Could you check a few things on this model? Use its own coordinates, in mm. Face numbers are marked on the shaded views. A direction names the side the tool comes from. Coordinates: 2 decimals unless noted, no trailing zeros. Write each loop counter-clockwise with the first axis right and the second up, starting at its lowest first coordinate (ties: lowest second). Pieces come first, ordered by that corner, then holes.
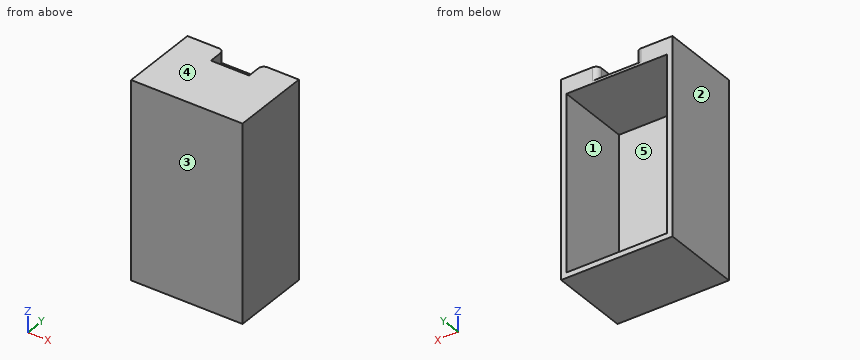
```python
from build123d import *

# Parameters (mm, degrees)
ESQUISSE1_W             = 210
ESQUISSE1_H             = 150
BOSS_EXTRU_1_DEPTH      = 370
ESQUISSE2_W             = 190
ESQUISSE2_H             = 330
ENL_V_MAT_EXTRU_1_DEPTH = 140
ESQUISSE6_W             = 72
ESQUISSE6_H             = 25
ENL_V_MAT_EXTRU_4_DEPTH = 35
ESQUISSE7_W             = 72
ESQUISSE7_H             = 20
ENL_V_MAT_EXTRU_5_DEPTH = 15
CONG_3_R                = 10
CONG_4_R                = 10
CONG_5_R                = 10


with BuildPart() as part:
    # Esquisse1 → Boss.-Extru.1 (new body)
    with BuildSketch(Plane.XY):
        with Locations((-54.477344992, -11.176470588)):
            Rectangle(ESQUISSE1_W, ESQUISSE1_H)
    extrude(amount=-BOSS_EXTRU_1_DEPTH)

    # Esquisse2 → Enlèv. mat.-Extru.1 (cut)
    with BuildSketch(Plane(origin=(0, 63.823529412, 0), x_dir=(1, 0, 0), z_dir=(0, 1, 0))):
        with Locations((-54.477344992, 195)):
            Rectangle(ESQUISSE2_W, ESQUISSE2_H)
    extrude(amount=-ENL_V_MAT_EXTRU_1_DEPTH, mode=Mode.SUBTRACT)

    # Esquisse6 → Enlèv. mat.-Extru.4 (cut)
    with BuildSketch(Plane(origin=(0, 63.823529412, 0), x_dir=(1, 0, 0), z_dir=(0, 1, 0))):
        with Locations((-54.477344992, 12.5)):
            Rectangle(ESQUISSE6_W, ESQUISSE6_H)
    extrude(amount=-ENL_V_MAT_EXTRU_4_DEPTH, mode=Mode.SUBTRACT)

    # Esquisse7 → Enlèv. mat.-Extru.5 (cut)
    with BuildSketch(Plane(origin=(0, 28.823529412, 0), x_dir=(1, 0, 0), z_dir=(0, 1, 0))):
        with Locations((-54.477344992, 15)):
            Rectangle(ESQUISSE7_W, ESQUISSE7_H)
    extrude(amount=-ENL_V_MAT_EXTRU_5_DEPTH, mode=Mode.SUBTRACT)

    # Congé3
    cong_3_edges = [part.edges().sort_by_distance(p)[0] for p in [
        (-90.477344992, 63.823529412, -12.5),
    ]]
    fillet(cong_3_edges, radius=CONG_3_R)

    # Congé4
    cong_4_edges = [part.edges().sort_by_distance(p)[0] for p in [
        (-18.477344992, 63.823529412, -12.5),
    ]]
    fillet(cong_4_edges, radius=CONG_4_R)

    # Congé5
    # the kernel refuses this fillet: 10 mm, written as the material it takes off along each edge
    with BuildSketch(Plane(origin=(-18.477344992, 28.823529412, -5), x_dir=(0, 0, 1), z_dir=(-1, 0, 0))) as cong_5_piece_1:
        with BuildLine():
            CenterArc((10, -8.660254038), CONG_5_R, 120, 60)
            Line((0, -8.660254038), (-0.2, -8.660254038))
            Line((-0.2, -8.660254038), (-0.2, 0))
            Line((-0.2, 0), (0, 0.2))
            ThreePointArc((0, 0.2), (2.5, 0.2), (4.9, 0.173205081))
            Line((4.9, 0.173205081), (5, 0))
        make_face()
    extrude(amount=72, mode=Mode.SUBTRACT)


solid = part.part
```
1. Please list where these lines run through material, in increasing order: line 1 along Z through (x, y) = (-132, 5.5); line 2 along X through (y, z) = (-4.5, -270.5); line 3 along Z through (x, y) = (-27, 24).
Verdict:
line 1: z = -370 to -360, -30 to 0
line 2: x = -159.48 to -149.48, 40.52 to 50.52
line 3: z = -370 to -360, -30 to -25, -4.23 to 0
2. I want a section at B-B on z = -138.5. Please give me the cut outline in (x, y), plus the area to 3 significant figures.
Verdict:
outline: (-159.48, -86.18) - (50.52, -86.18) - (50.52, 63.82) - (40.52, 63.82) - (40.52, -76.18) - (-149.48, -76.18) - (-149.48, 63.82) - (-159.48, 63.82) - close
area: 4,900 mm2
3. On a 3-axis mill with a long thin cutter (end or side, diameter ignored), from which of +Z, -Z, +X, -X, +Y, -Y can I reach the whole of each face in a straight line? I mean the marked faces 4 and 5. Say none if no direction works.
Verdict:
face 4: +Z, +X, -X, +Y, -Y
face 5: +Y
4. I want a section at C-C on x = -108. Please give me the cut outline in (y, z).
Verdict:
outline: (-86.18, -370) - (63.82, -370) - (63.82, -360) - (-76.18, -360) - (-76.18, -30) - (63.82, -30) - (63.82, 0) - (-86.18, 0) - close
5. For pin 1 (10 mm diameter, centred on x = -71, z = -18.5, fed in from +Y); pin 2 (1.5 mm diameter, centred on x = -17, z = -234.5, fed in from +Y); pin 3 (15 mm diameter, centred on x = -72, y = 47, fed in from +Z), each with a flat end and sliding along its axis, tell me the tip position at first contact or that it passes through.
Verdict:
pin 1: stops at y = 13.82
pin 2: stops at y = -76.18
pin 3: stops at z = -25
6. If we mould it in two halves opening along X, with no side actions, what happens to the marked faces 1, 2 and 3? For each: pulls with the +X half, pulls with the -X half, needs draft (parallel to the pull), parting line crosses it, or undercut.
Verdict:
face 1: undercut
face 2: pulls with the -X half
face 3: needs draft
7. I want a section at D-D on y = 35. Please give me the cut outline in (x, z).
Verdict:
outline: (-159.48, -370) - (50.52, -370) - (50.52, 0) - (-18.48, 0) - (-18.48, -25) - (-90.48, -25) - (-90.48, 0) - (-159.48, 0) - close; hole (-149.48, -360) - (40.52, -360) - (40.52, -30) - (-149.48, -30) - close
8. I want a section at A-A on y = -27. Please give me the cut outline in (x, z).
Verdict:
outline: (-159.48, -370) - (50.52, -370) - (50.52, 0) - (-159.48, 0) - close; hole (-149.48, -360) - (40.52, -360) - (40.52, -30) - (-149.48, -30) - close
